CAD build for the part. Positions are in the model's coordinates, mm. Give positions to 0.01 mm unless a question says otherwise; leave off trailing zeros. Write each loop counter-clockwise with the first axis right and the second up, starting at its lowest first coordinate (ties: lowest second). Pieces come first, ordered by that corner, then holes. Notation, with made-up numbers: (-8.5, -21) -> (46.5, -21) arc R32 cw to (46.5, 5) -> close; hole circle Ø2 at (48.25, 35.25). An arc over 180 degrees is marked (long way). Answer in a Markdown table with one row per item. Add a question column.
```python
from build123d import *

# Parameters (mm, degrees)
BOSS_EXTRUDE1_DEPTH = 2.5
SKETCH2_R           = 1.5
CUT_EXTRUDE1_DEPTH  = 2.5
FILLET1_R           = 1.5


with BuildPart() as part:
    # Sketch1 → Boss-Extrude1 (new body)
    with BuildSketch(Plane(origin=(0, 0, 0), x_dir=(1, 0, 0), z_dir=(0, 1, 0))):
        with BuildLine():
            Line((-233.299741314, 67.325465398), (-233.299741314, -21.174534602))
            ThreePointArc((-233.299741314, -21.174534602), (-231.292382001, -25.52072868), (-226.799741314, -27.174534602))
            Line((-226.799741314, -27.174534602), (-221.799741314, -27.174534602))
            Line((-221.799741314, -27.174534602), (-221.799741314, -29.174534602))
            Line((-221.799741314, -29.174534602), (-150.799741314, -29.174534602))
            Line((-150.799741314, -29.174534602), (-150.799741314, -27.174534602))
            Line((-150.799741314, -27.174534602), (-145.799741314, -27.174534602))
            ThreePointArc((-145.799741314, -27.174534602), (-141.307100627, -25.52072868), (-139.299741314, -21.174534602))
            Line((-139.299741314, -21.174534602), (-139.299741314, 67.325465398))
            Line((-139.299741314, 67.325465398), (-139.299741314, 99.825465398))
            Line((-139.299741314, 99.825465398), (-145.799741314, 99.825465398))
            Line((-145.799741314, 99.825465398), (-145.799741314, 67.325465398))
            Line((-145.799741314, 67.325465398), (-145.799741314, -16.174534602))
            ThreePointArc((-145.799741314, -16.174534602), (-147.264207408, -19.710068508), (-150.799741314, -21.174534602))
            Line((-150.799741314, -21.174534602), (-221.799741314, -21.174534602))
            ThreePointArc((-221.799741314, -21.174534602), (-225.33527522, -19.710068508), (-226.799741314, -16.174534602))
            Line((-226.799741314, -16.174534602), (-226.799741314, 67.325465398))
            Line((-226.799741314, 67.325465398), (-226.799741314, 99.825465398))
            Line((-226.799741314, 99.825465398), (-233.299741314, 99.825465398))
            Line((-233.299741314, 99.825465398), (-233.299741314, 67.325465398))
        make_face()
    extrude(amount=BOSS_EXTRUDE1_DEPTH)

    # Sketch2 → Cut-Extrude1 (cut)
    with BuildSketch(Plane(origin=(0, 2.5, 0), x_dir=(1, 0, 0), z_dir=(0, 1, 0))):
        with Locations((-230.049741314, 7.325465398)):
            Circle(SKETCH2_R)
        with Locations((-142.549741314, 7.325465398)):
            Circle(SKETCH2_R)
        with Locations((-230.049741314, 31.325465398)):
            Circle(SKETCH2_R)
        with Locations((-230.049741314, 55.325465398)):
            Circle(SKETCH2_R)
        with Locations((-230.049741314, 43.325465398)):
            Circle(SKETCH2_R)
        with Locations((-230.049741314, 19.325465398)):
            Circle(SKETCH2_R)
        with Locations((-230.049741314, -4.674534602)):
            Circle(SKETCH2_R)
        with Locations((-142.549741314, -4.674534602)):
            Circle(SKETCH2_R)
        with Locations((-142.549741314, 19.325465398)):
            Circle(SKETCH2_R)
        with Locations((-142.549741314, 31.325465398)):
            Circle(SKETCH2_R)
        with Locations((-142.549741314, 43.325465398)):
            Circle(SKETCH2_R)
        with Locations((-142.549741314, 55.325465398)):
            Circle(SKETCH2_R)
        with Locations((-230.049741314, -16.674534602)):
            Circle(SKETCH2_R)
        with Locations((-142.549741314, -16.674534602)):
            Circle(SKETCH2_R)
        with Locations((-216.854480823, -25.174534602)):
            Circle(SKETCH2_R)
        with Locations((-155.745001805, -25.174534602)):
            Circle(SKETCH2_R)
        with Locations((-230.049741314, 67.325465398)):
            Circle(SKETCH2_R)
        with Locations((-142.549741314, 67.325465398)):
            Circle(SKETCH2_R)
        with Locations((-230.049741314, 79.325465398)):
            Circle(SKETCH2_R)
        with Locations((-142.549741314, 79.325465398)):
            Circle(SKETCH2_R)
        with Locations((-230.049741314, 91.325465398)):
            Circle(SKETCH2_R)
        with Locations((-142.549741314, 91.325465398)):
            Circle(SKETCH2_R)
    extrude(amount=-CUT_EXTRUDE1_DEPTH, mode=Mode.SUBTRACT)

    # Fillet1
    fillet1_edges = [part.edges().sort_by_distance(p)[0] for p in [
        (-145.799741314, 1.25, -99.825465398),
        (-139.299741314, 1.25, -99.825465398),
        (-233.299741314, 1.25, -99.825465398),
        (-226.799741314, 1.25, -99.825465398),
    ]]
    fillet(fillet1_edges, radius=FILLET1_R)


solid = part.part
```
Item 1: Mould opens along Z. For faces 1 (the face through (-141.164, 1.268, 17.249)), 2 (the face through (-141.164, 1.268, -42.751)), 3 (the face through (-226.8, 1, -40)), 4 (the face through (-143, 1, -99.825)) say: released by +Z, released by -Z, zero draft, split by the parting line, or undercut.
Item 2: Drop flat-ended pins along their axis: pin 1 Ø1.8 at (x, z) = (-216.85, 25.17) entering from +Y; pin 2 Ø1 at (x, y) = (-160, 1) entering from -Z. Give the stop position or say it passes through.
Item 3: Slice it at A-A, the plane z = -61. List the corners of the cut face in (x, y).
Item 4: Probe L1, parallel to X at y = 1.15, z = -79; L2, parallel to X at y = 2.1, z = 17; L3, parallel to X at y = 1.1, z = -93.5. List the from-to ranges inside material, lowest first. Write a range as from..to.
Item 5: Slice it at B-B, the plane x = -192.5. List the corners of the cut face in (y, z), then the cut area to 3 significant figures.
Item 6: Slice it at C-C, the plane y = 2. State how many separate pieces and enclosed holes the cut face has, then the cut area to 3 significant figures.
Answer key:
| question | item | result |
|---|---|---|
| 1 | face 1 | undercut |
| 1 | face 2 | undercut |
| 1 | face 3 | zero draft |
| 1 | face 4 | released by -Z |
| 2 | pin 1 | passes through |
| 2 | pin 2 | stops at z = 21.17 |
| 3 | outline | (-233.3, 0) -> (-226.8, 0) -> (-226.8, 2.5) -> (-233.3, 2.5) -> close; (-145.8, 0) -> (-139.3, 0) -> (-139.3, 2.5) -> (-145.8, 2.5) -> close |
| 4 | L1 | x = -233.3..-231.51, -228.59..-226.8, -145.8..-144.01, -141.09..-139.3 |
| 4 | L2 | x = -233.3..-231.51, -228.59..-226.73, -145.87..-144.01, -141.09..-139.3 |
| 4 | L3 | x = -233.3..-226.8, -145.8..-139.3 |
| 5 | outline | (0, 21.17) -> (2.5, 21.17) -> (2.5, 29.17) -> (0, 29.17) -> close |
| 5 | area | 20.0 mm² |
| 6 | separate pieces | 1 |
| 6 | enclosed holes | 22 |
| 6 | area | 2,120 mm² |
